Check sheet for the modelled part. Datum: model origin and axes. Units: mm. Give positions to 0.01 mm unless a question says otherwise; leave off trailing zeros. Loops run counter-clockwise (first coordinate to the right, second up) from the corner with the lowest first, then second, coordinate; pieces in that order, holes last. Notation, with made-up numbers: (-8.75, -8) -> (40.25, -8) arc R25 ccw to (40.25, 25) -> close; hole circle Ø6 at (-37, 56). An arc over 180 degrees is marked (long way). Write each question's results on one line, items separated by ' | '. Start each with the question number.
Item 1: Cross-section at C-C on x = 38. Enter the section's corners in (y, z).
Item 2: Scan lines: line 1 along X through (y, z) = (7, 2.8); line 2 along Y through (x, z) = (-38.5, 1.2); line 3 along X through (y, z) = (11, 0.5). Record each from-to range of solid material in increasing order.
Item 3: Cross-section at B-B on y = 12.5. Enter the section's corners in (x, z), then the cut area to 3 significant figures.
Item 4: Cross-section at D-D on z = 3.6. State how many separate pieces and enclosed holes the cut face has, then the cut area to 3 significant figures.
Item 5: Cross-section at A-A on x = 3.5. Enter the section's corners in (y, z), then the cut area to 3 significant figures.
Item 6: Gauge pin test, flat ends, axial feed: pin 1 Ø2.5 at (x, z) = (-4.5, 3) entering from -Y; pin 2 Ø2 at (x, z) = (40.5, 3) entering from +Y; pin 3 Ø1.5 at (x, z) = (-41.5, 2) entering from +Y. Record the tip position at first contact, or that the pin passes through.
from build123d import *

# Parameters (mm, degrees)
F0_R     = 55.5625
F2_DEPTH = 4.7625
F1_R     = 9.525
F3_DEPTH = 4.7625
F5_R     = 14.2875
F6_DEPTH = 25.4


with BuildPart() as f2:
    # F0 (on Top) → F2 (new body)
    with BuildSketch(Plane.XY):
        Circle(F0_R)
    extrude(amount=F2_DEPTH)

    # F1 (on Top) → F3 (cut, through all)
    with BuildSketch(Plane.XY):
        with Locations((-45.8453687481, -31.3909791278)):
            Circle(F1_R)
        with Locations((0, 55.5625)):
            Circle(F1_R)
        with Locations((45.8453687481, -31.3909791278)):
            Circle(F1_R)
    extrude(amount=F3_DEPTH, mode=Mode.SUBTRACT)

    # F5 (on face) → F6 (cut)
    with BuildSketch(Plane(origin=(0, 0, 0), x_dir=(1, 0, 0), z_dir=(0, 0, -1))):
        with Locations((-28.0854459631, -14.8077758308)):
            Circle(F5_R)
        with Locations((28.0854459631, -14.8077758308)):
            Circle(F5_R)
        Polygon((16.7959635843, 34.0323393857), (0, 46.2353212285), (-16.7959635843, 34.0323393857), (-10.3804763689, 14.2875), (10.3804763689, 14.2875), align=None)
    extrude(amount=-F6_DEPTH, mode=Mode.SUBTRACT)


solid = f2.part
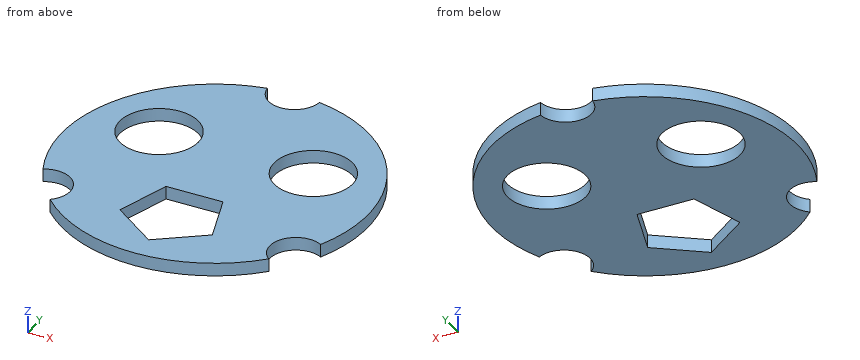
Answer sheet:
1) outline: (-40.54, 0) -> (-36.79, 0) -> (-36.79, 4.76) -> (-40.54, 4.76) -> close; (-25.99, 0) -> (4.52, 0) -> (4.52, 4.76) -> (-25.99, 4.76) -> close; (25.1, 0) -> (40.54, 0) -> (40.54, 4.76) -> (25.1, 4.76) -> close
2) line 1: x = -55.12 to -40.05, -16.12 to 16.12, 40.05 to 55.12 | line 2: y = -40.06 to -37.45, -25.33 to 5.03, 24.59 to 40.06 | line 3: x = -54.46 to -41.86, -14.31 to 14.31, 41.86 to 54.46
3) outline: (-54.14, 0) -> (-42.19, 0) -> (-42.19, 4.76) -> (-54.14, 4.76) -> close; (-13.99, 0) -> (13.99, 0) -> (13.99, 4.76) -> (-13.99, 4.76) -> close; (42.19, 0) -> (54.14, 0) -> (54.14, 4.76) -> (42.19, 4.76) -> close | area: 247 mm²
4) separate pieces: 1 | enclosed holes: 3 | area: 7,260 mm²
5) outline: (-55.45, 0) -> (-43.69, 0) -> (-43.69, 4.76) -> (-55.45, 4.76) -> close; (-14.29, 0) -> (46.7, 0) -> (46.7, 4.76) -> (-14.29, 4.76) -> close | area: 346 mm²
6) pin 1: stops at y = -55.47 | pin 2: stops at y = 39.08 | pin 3: stops at y = 37.77
